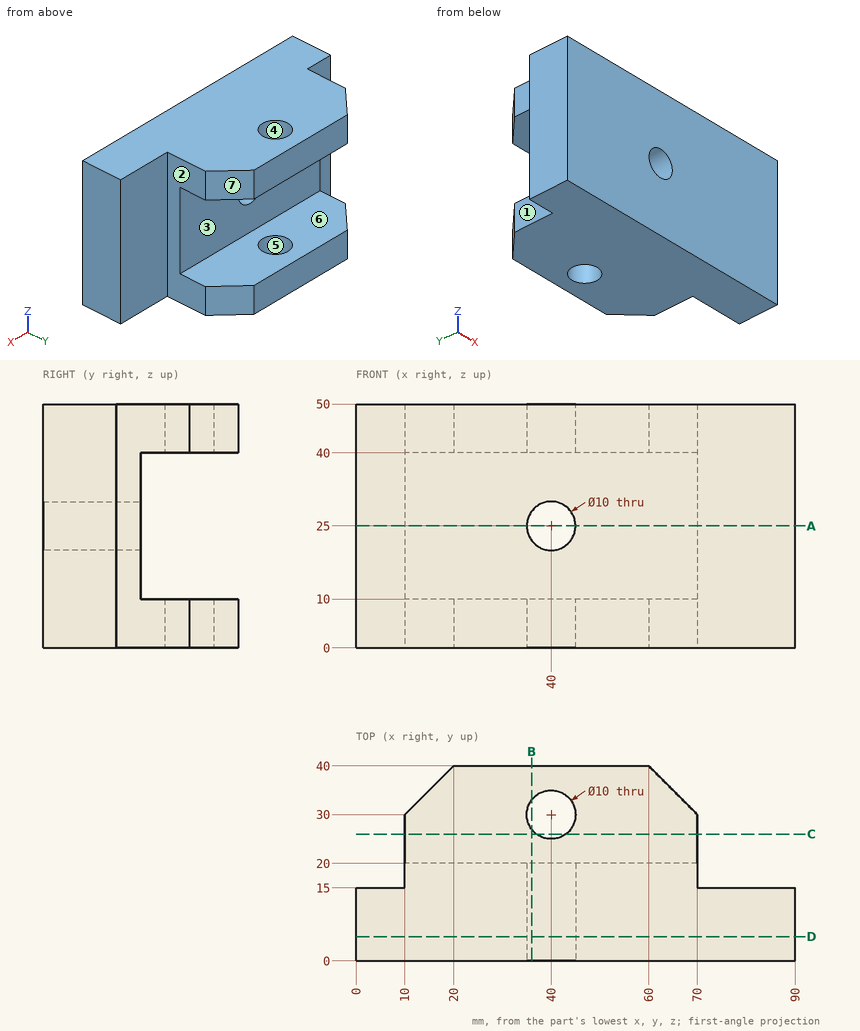
Drawing for the job (mm, zero at the part's lowest x, y, z). A direction names the side the tool comes from. Round coordinates to 2 decimals unless told otherwise and drop trailing zeros. Write each loop counter-clockwise with the first axis right and the second up, starting at its lowest first coordinate (ties: lowest second). Pieces come first, ordered by that corner, then holes. Notation, with made-up numbers: M 84,24 L 92,24 A21 cw 92,47 Z; hole C 26,-6 d2. An arc over 180 degrees is marked long. One line per question, with ' | ' between items.
1. Pin check, flat tips, straight feed: pin 1 Ø10 at (y, z) = (28.5, 29) entering from +X; pin 2 Ø6 at (x, z) = (79, 30.5) entering from +Y; pin 3 Ø12 at (y, z) = (23.5, 22.5) entering from -X; pin 4 Ø13 at (x, z) = (40, 25) entering from +Y. Stop position of each tip, or through.
Working result:
pin 1: through | pin 2: y = 15 | pin 3: x = 10 | pin 4: y = 20
2. Mould opens along Y. For the marked faces 4, 5, 6 and 7 say: pulls with the +Y half, pulls with the -Y half, needs draft (parallel to the pull), parting line crosses it, or undercut.
Working result:
face 4: undercut | face 5: undercut | face 6: needs draft | face 7: pulls with the +Y half
3. Which spindle directions (+Z, -Z, +X, -X, +Y, -Y) get a long thin tool onto all of the face, cutting with end or side? Do the marked faces 1, 2 and 3. Say none if no direction does.
Working result:
face 1: +Z, -Z, -X, +Y | face 2: +Z, -Z, +X, +Y | face 3: +X, -X, +Y
4. Cut at A-A on z = 25. Write the cut outline in (x, y).
Working result:
outline: M 0,0 L 35,0 L 35,20 L 10,20 L 10,15 L 0,15 Z; M 45,0 L 90,0 L 90,15 L 70,15 L 70,20 L 45,20 Z
5. Probe L1, parallel to Z at x = 17, y = 32.5; L2, parallel to X at y = 30, z = 47; L3, parallel to Z at x = 40, y = 4.5. List the from-to ranges inside material, lowest first. Write a range as from..to.
Working result:
L1: 0..10, 40..50 | L2: 10..35, 45..70 | L3: 0..20, 30..50
6. Cut at B-B on x = 36. Write the cut outline in (y, z), and give its area (3 significant figures).
Working result:
outline: M 0,0 L 27,0 L 27,10 L 20,10 L 20,22 L 0,22 Z; M 0,28 L 20,28 L 20,40 L 27,40 L 27,50 L 0,50 Z; M 33,0 L 40,0 L 40,10 L 33,10 Z; M 33,40 L 40,40 L 40,50 L 33,50 Z | area: 1,160 mm2
7. Cut at C-C on y = 26. Write the cut outline in (x, z), and give its area (3 significant figures).
Working result:
outline: M 10,0 L 37,0 L 37,10 L 10,10 Z; M 10,40 L 37,40 L 37,50 L 10,50 Z; M 43,0 L 70,0 L 70,10 L 43,10 Z; M 43,40 L 70,40 L 70,50 L 43,50 Z | area: 1,080 mm2
8. Cut at D-D on y = 5. Write the cut outline in (x, z), and give its area (3 significant figures).
Working result:
outline: M 0,0 L 90,0 L 90,50 L 0,50 Z; hole C 40,25 d10 | area: 4,420 mm2
